from build123d import *

# Parameters (mm, degrees)
BOSS_EXTRUDE1_DEPTH = 5
SKETCH2_R           = 5
BOSS_EXTRUDE2_DEPTH = 5
SKETCH3_R           = 5
CUT_EXTRUDE1_DEPTH  = 28.386127875


with BuildPart() as part:
    # Sketch1 → Boss-Extrude1 (new body)
    with BuildSketch(Plane(origin=(0, 0, 0), x_dir=(1, 0, 0), z_dir=(0, 1, 0))):
        with BuildLine():
            Line((-15, 10), (15, 10))
            ThreePointArc((15, 10), (25, 0), (15, -10))
            Line((15, -10), (-15, -10))
            ThreePointArc((-15, -10), (-25, 0), (-15, 10))
        make_face()
    extrude(amount=BOSS_EXTRUDE1_DEPTH)

    # Sketch2 → Boss-Extrude2 (add)
    with BuildSketch(Plane(origin=(0, 5, 0), x_dir=(1, 0, 0), z_dir=(0, 1, 0))):
        with Locations(Location((15, 0, 0), (0, 0, 270))):
            Circle(SKETCH2_R)
    extrude(amount=BOSS_EXTRUDE2_DEPTH)

    # Sketch3 → Cut-Extrude1 (cut, through all)
    with BuildSketch(Plane(origin=(0, 5, 0), x_dir=(1, 0, 0), z_dir=(0, 1, 0))):
        with Locations(Location((-15, 0, 0), (0, 0, 270))):
            Circle(SKETCH3_R)
    extrude(amount=-CUT_EXTRUDE1_DEPTH, mode=Mode.SUBTRACT)


solid = part.part
Could you check a few things on this model? Use its own coordinates, in mm. Give positions to 0.01 mm unless a question says otherwise; leave off trailing zeros. Order: outer loops, then holes, each group sorted by start corner. A loop starts at its lowest first (then second) coordinate and runs counter-clockwise, first axis right, second up. Notation, with made-up numbers: (-0.5, 89.5) -> (23.5, 89.5) arc R17 cw to (23.5, 95.5) -> close; hole circle Ø9 at (-23.5, 88.25). An arc over 180 degrees is marked (long way). Answer in a Markdown table with one row per item. Add a question column.
Item 1: We'd pull the mould along X, two halves only. Please class faces 1 (the cylindrical face through (10.12, 7.46, -1.08)), 2 (the flat face through (0, 5, 0)), 3 (the cylindrical face through (-19.88, 2.54, -1.08)): pulls with the +X half, pulls with the -X half, needs draft (parallel to the pull), parting line crosses it, or undercut.
Item 2: I'm going to push flat-ended pins straight in: P1, Ø1.5, axis at y = 8.5, z = 1.5, coming from the -X side; P2, Ø1, axis at x = 4, z = 7, coming from the -Y side; P3, Ø2, axis at y = 2.5, z = -2, coming from the -X side; P4, Ø6, axis at y = 8.5, z = -5, coming from the -X side. Where does each tip first touch, or does it pass through?
Item 3: Imagine slicing it at D-D (x = 6). List the corners of the cut face in (y, z) for me.
Item 4: Imagine slicing it at A-A (z = 0). List the corners of the cut face in (x, y) for me, and give its area (3 significant figures).
Item 5: Imagine slicing it at B-B (y = 1.75). List the corners of the cut face in (x, z) for me.
Item 6: Imagine slicing it at C-C (z = -4.5). List the corners of the cut face in (x, y) for me, and give its area (3 significant figures).
Item 7: Please list where these lines run through material, in increasing order: probe 1 along X at (y, z) = (1.8, 0); probe 2 along Y at (x, z) = (-4, -7); probe 3 along X at (y, z) = (8, 0).
Result:
| question | item | result |
|---|---|---|
| 1 | face 1 | parting line crosses it |
| 1 | face 2 | needs draft |
| 1 | face 3 | undercut |
| 2 | P1 | x = 10.06 |
| 2 | P2 | y = 0 |
| 2 | P3 | x = -24.95 |
| 2 | P4 | x = 10.42 |
| 3 | outline | (0, -10) -> (5, -10) -> (5, 10) -> (0, 10) -> close |
| 4 | outline | (-25, 0) -> (-20, 0) -> (-20, 5) -> (-25, 5) -> close; (-10, 0) -> (25, 0) -> (25, 5) -> (20, 5) -> (20, 10) -> (10, 10) -> (10, 5) -> (-10, 5) -> close |
| 4 | area | 250 mm2 |
| 5 | outline | (-15, -10) -> (15, -10) arc R10 ccw to (15, 10) -> (-15, 10) arc R10 ccw to start; hole circle Ø10 at (-15, 0) |
| 6 | outline | (-23.93, 0) -> (-17.18, 0) -> (-17.18, 5) -> (-23.93, 5) -> close; (-12.82, 0) -> (23.93, 0) -> (23.93, 5) -> (17.18, 5) -> (17.18, 10) -> (12.82, 10) -> (12.82, 5) -> (-12.82, 5) -> close |
| 6 | area | 239 mm2 |
| 7 | probe 1 | -25 to -20, -10 to 25 |
| 7 | probe 2 | 0 to 5 |
| 7 | probe 3 | 10 to 20 |
